Model file for the job. Use its own axes, mm. Round coordinates to 2 decimals unless told otherwise and drop trailing zeros. Loops run counter-clockwise (first coordinate to the right, second up) from the corner with the lowest first, then second, coordinate; pieces in that order, holes last. Notation, with made-up numbers: M 30.25,71 L 70.25,71 A15 ccw 70.25,79 Z; hole C 21,11 d9. An arc over 180 degrees is marked long. Answer in a Markdown table with one row per item.
from build123d import *

# Parameters (mm, degrees)
SKETCH_1_W          = 20
SKETCH_1_H          = 12
SKETCH_1_R          = 3.25
SKETCH_1_R_2        = 1.65
EXTRUDE_1_DEPTH     = 7.5
SKETCH_3_R          = 1.4
CUT_EXTRUDE_1_DEPTH = 15
FILLET_1_R          = 1


with BuildPart() as part:
    # 草图1 → 凸台-拉伸1 (new, symmetric)
    with BuildSketch(Plane(origin=(0, 0, 0), x_dir=(1, 0, 0), z_dir=(0, 1, 0))):
        Rectangle(SKETCH_1_W, SKETCH_1_H)
        with Locations(Location((0, 0, 0), (0, 0, 270))):
            Circle(SKETCH_1_R, mode=Mode.SUBTRACT)
        with Locations(Location((-7, 0, 0), (0, 0, 270))):
            Circle(SKETCH_1_R_2, mode=Mode.SUBTRACT)
        with Locations(Location((7, 0, 0), (0, 0, 270))):
            Circle(SKETCH_1_R_2, mode=Mode.SUBTRACT)
    extrude(amount=EXTRUDE_1_DEPTH, both=True)

    # 草图3 → 切除-拉伸1 (cut)
    with BuildSketch(Plane(origin=(0, 0, -6), x_dir=(-1, 0, 0), z_dir=(0, 0, -1))):
        with Locations((0, 4)):
            Circle(SKETCH_3_R)
        with Locations((0, -4)):
            Circle(SKETCH_3_R)
    extrude(amount=-CUT_EXTRUDE_1_DEPTH, mode=Mode.SUBTRACT)

    # 圆角1
    fillet_1_edges = [part.edges().sort_by_distance(p)[0] for p in [
        (-10, 7.5, 0),
        (0, 7.5, 6),
        (10, 7.5, 0),
        (0, -7.5, 6),
        (-10, -7.5, 0),
        (0, -7.5, -6),
        (10, -7.5, 0),
        (10, 0, 6),
        (-10, 0, 6),
        (-10, 0, -6),
        (10, 0, -6),
        (0, 7.5, -6),
    ]]
    fillet(fillet_1_edges, radius=FILLET_1_R)


solid = part.part
1. Wall check: probe 1 along X at (y, z) = (-3.75, 0); probe 2 along Y at (x, z) = (0, -3.55); probe 3 along X at (y, z) = (-4, -4). Give the ranges that are in metal, low to high.
Verdict:
| item | result |
|---|---|
| probe 1 | x = -10 to -8.65, -5.35 to -3.25, 3.25 to 5.35, 8.65 to 10 |
| probe 2 | y = -7.5 to -5.4, -2.6 to 2.6, 5.4 to 7.5 |
| probe 3 | x = -10 to -1.4, 1.4 to 10 |
2. Saw through at B-B (z = 0). Write the cut outline in (x, y), and give its area (3 significant figures).
Verdict:
| item | result |
|---|---|
| outline | M -10,-6.5 A1 ccw -9,-7.5 L -8.65,-7.5 L -8.65,7.5 L -9,7.5 A1 ccw -10,6.5 Z; M -5.35,-7.5 L -3.25,-7.5 L -3.25,7.5 L -5.35,7.5 Z; M 3.25,-7.5 L 5.35,-7.5 L 5.35,7.5 L 3.25,7.5 Z; M 8.65,-7.5 L 9,-7.5 A1 ccw 10,-6.5 L 10,6.5 A1 ccw 9,7.5 L 8.65,7.5 Z |
| area | 103 mm² |
3. Pin check, flat tip, straight feed: pin 1 (4 mm diameter, centred on x = 7, z = 0, fed in from +Y). Stop position of the tip, or through.
Verdict:
| item | result |
|---|---|
| pin 1 | stops at y = 7.5 |
4. Saw through at C-C (x = -7). Write the cut outline in (y, z), and give its area (3 significant figures).
Verdict:
| item | result |
|---|---|
| outline | M -7.5,-5 A1 ccw -6.5,-6 L 6.5,-6 A1 ccw 7.5,-5 L 7.5,-1.65 L -7.5,-1.65 Z; M -7.5,1.65 L 7.5,1.65 L 7.5,5 A1 ccw 6.5,6 L -6.5,6 A1 ccw -7.5,5 Z |
| area | 130 mm² |
5. Saw through at A-A (y = -4). Write the cut outline in (x, z).
Verdict:
| item | result |
|---|---|
| outline | M -10,-5 A1 ccw -9,-6 L -1.4,-6 L -1.4,-2.93 A3.25 cw -1.4,2.93 L -1.4,6 L -9,6 A1 ccw -10,5 Z; M 1.4,-6 L 9,-6 A1 ccw 10,-5 L 10,5 A1 ccw 9,6 L 1.4,6 L 1.4,2.93 A3.25 cw 1.4,-2.93 Z; hole C -7,0 d3.3; hole C 7,0 d3.3 |
6. Saw through at D-D (z = 4). Write the cut outline in (x, y), and give its area (3 significant figures).
Verdict:
| item | result |
|---|---|
| outline | M -10,-6.5 A1 ccw -9,-7.5 L 9,-7.5 A1 ccw 10,-6.5 L 10,6.5 A1 ccw 9,7.5 L -9,7.5 A1 ccw -10,6.5 Z; hole C 0,-4 d2.8; hole C 0,4 d2.8 |
| area | 287 mm² |
7. Mould opens along X. For faces 1 (the cylindrical face through (1.4, -3.94, 4.45)), 2 (the flat face through (0, 0, -6)), 3 (the cylindrical face through (9.699, -0.091, -5.715)) say: +X half, -X half, draft (parallel to the pull), parting line (faces both ways), or undercut.
Verdict:
| item | result |
|---|---|
| face 1 | undercut |
| face 2 | draft |
| face 3 | +X half |
